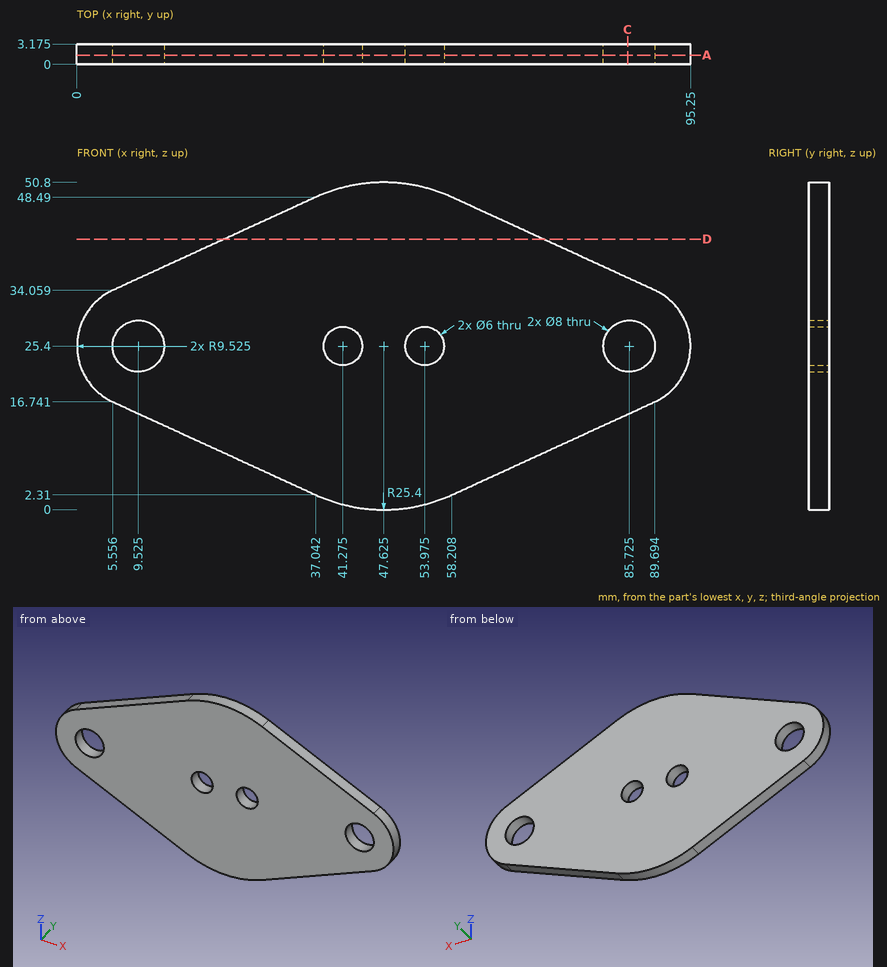
Answer from the drawing. Dimensions are ordinates in mm from the lowest x, y and z of the part. Round coordinates to 2 decimals unless told otherwise and drop trailing zeros. Loops run counter-clockwise (first coordinate to the right, second up) from the corner with the lowest first, then second, coordinate; pieces in that order, holes last. Notation, with made-up numbers: M -7,32.5 L 7,32.5 A15 cw 7,41.5 Z; hole C -3.75,38 d1. An arc over 180 degrees is marked long. One line per question, with ' | ' between items. Start each with the question number.
(1) Flat-ended cylindrical pins translate along their axes: pin 1 Ø7 at (x, z) = (9.525, 25.4) entering from -Y; pin 2 Ø1 at (y, z) = (2, 34) entering from -X (1 decimal). Find the tip coordinate at first contact, or state that the pin passes through.
(2) Find the intervals of material crossed by line 1 (X direction, y = 0.1, z = 22) (1 decimal); line 2 (X direction, y = 1.25, z = 28.5) (1 decimal); line 3 (Z direction, x = 51.5, y = 2.5) (1 decimal), in increasing order.
(3) A cutting plane is placed at C-C on x = 85.5. Write down the section's boundary in (y, z) (1 decimal).
(4) A cutting plane is placed at D-D on z = 42. Write down the section's boundary in (x, y) (1 decimal).
(5) A cutting plane is placed at A-A on y = 1.45. Give the number of separate pieces and of enclosed holes in the cut face, plus the area to 3 significant figures.
Geometry check:
1) pin 1: passes through | pin 2: stops at x = 4.5
2) line 1: x = 0.6 to 7.4, 11.6 to 83.6, 87.8 to 94.6 | line 2: x = 0.5 to 7, 12.1 to 83.2, 88.3 to 94.7 | line 3: z = 0.3 to 23.7, 27.1 to 50.5
3) outline: M 0,14.8 L 3.2,14.8 L 3.2,21.4 L 0,21.4 Z; M 0,29.4 L 3.2,29.4 L 3.2,36 L 0,36 Z
4) outline: M 22.9,0 L 72.4,0 L 72.4,3.2 L 22.9,3.2 Z
5) separate pieces: 1 | enclosed holes: 4 | area: 3,020 mm²
